Could you check a few things on this model? Use its own coordinates, in mm. Give positions to 0.01 mm unless a question says otherwise; leave off trailing zeros. Order: outer loops, then holes, each group sorted by start corner. A loop starts at its lowest first (then second) coordinate and runs counter-clockwise, first axis right, second up. Notation, with made-up numbers: M 57,-16 L 107,-16 A22 cw 107,0 Z; hole C 29.25,21 d10. An arc over 180 degrees is marked long. Answer in a Markdown table with one row per item. Add a question column.
```python
from build123d import *

# Parameters (mm, degrees)
EXTRUDE_1_DEPTH          = 3
SKETCH_2_R               = 37.6
CUT_EXTRUDE_1_DEPTH      = 3
SKETCH_1_4_R             = 2.7
CUT_EXTRUDE_5_DEPTH      = 10
PATTERN_CIRCULAR_2_COUNT = 4


with BuildPart() as part:
    # Sketch 1 → Extrude 1 (new body)
    with BuildSketch(Plane(origin=(0, 0, 0), x_dir=(1, 0, 0), z_dir=(0, 1, 0))):
        with BuildLine():
            Line((-49, 45), (-49, -45))
            ThreePointArc((-49, -45), (-47.828427125, -47.828427125), (-45, -49))
            Line((-45, -49), (45, -49))
            ThreePointArc((45, -49), (47.828427125, -47.828427125), (49, -45))
            Line((49, -45), (49, 45))
            ThreePointArc((49, 45), (47.828427125, 47.828427125), (45, 49))
            Line((45, 49), (-45, 49))
            ThreePointArc((-45, 49), (-47.828427125, 47.828427125), (-49, 45))
        make_face()
    extrude(amount=EXTRUDE_1_DEPTH)

    # Sketch 2 → Cut-Extrude 1 (cut)
    with BuildSketch(Plane(origin=(0, 3, 0), x_dir=(1, 0, 0), z_dir=(0, 1, 0))):
        with Locations(Location((0, 0, 0), (0, 0, 270))):
            Circle(SKETCH_2_R)
    extrude(amount=-CUT_EXTRUDE_1_DEPTH, mode=Mode.SUBTRACT)

    # Sketch 1_4 → Cut-Extrude 5 (cut)
    with BuildSketch(Plane(origin=(0, 0, 0), x_dir=(1, 0, 0), z_dir=(0, 1, 0))):
        with Locations(Location((45, -45, 0), (0, 0, 270))):
            Circle(SKETCH_1_4_R)
    cut_extrude_5 = extrude(amount=CUT_EXTRUDE_5_DEPTH, mode=Mode.SUBTRACT)

    # Pattern Circular 2: Cut-Extrude 5 ×4 about axis
    pattern_circular_2_axis = Axis((0, 0, 0), (0, 1, 0))
    for i in range(1, PATTERN_CIRCULAR_2_COUNT):
        add(cut_extrude_5.rotate(pattern_circular_2_axis, i * 360 / PATTERN_CIRCULAR_2_COUNT), mode=Mode.SUBTRACT)


solid = part.part
```
1. Suppose I cut it at A-A on y = 1.1. List the corners of the cut face in (x, z) for me, plus the area to 3 significant figures.
2. Suppose I cut it at C-C on x = 0. List the corners of the cut face in (y, z) for me.
3. Suppose I cut it at B-B on z = 0. List the corners of the cut face in (x, y) for me, plus the area to 3 significant figures.
4. If I drill on line 1 along Z through (x, y) = (45, 1.45); line 2 along Z through (x, y) = (0.5, 0.25), over which ranges is the centre line in solid material (lowest first)? Write a range as [from, to].
5. Thinking about a two-plate mould opening in X: for faces 1 (the flat face through (-1, 1, 49)), 2 (the flat face through (-49, 1, -1)), 3 (the cylindrical face through (-47.575, 1.479, 45.811)), 4 (the cylindrical face through (47.859, 1.479, -47.797)), which applies, pulls with the +X half, pulls with the -X half, needs draft (parallel to the pull), parting line crosses it, or undercut?
6. Will these pins go through, and if not, where does the flat tip stop? P1, Ø10, axis at x = 34.5, z = 12, coming from the +Y side; P2, Ø4.5, axis at x = -45, z = -45, coming from the +Y side.
Findings below:
| question | item | result |
|---|---|---|
| 1 | outline | M -49,-45 A4 ccw -45,-49 L 45,-49 A4 ccw 49,-45 L 49,45 A4 ccw 45,49 L -45,49 A4 ccw -49,45 Z; hole C -45,-45 d5.4; hole C -45,45 d5.4; hole C 0,0 d75.2; hole C 45,-45 d5.4; hole C 45,45 d5.4 |
| 1 | area | 5,060 mm2 |
| 2 | outline | M 0,-49 L 3,-49 L 3,-37.6 L 0,-37.6 Z; M 0,37.6 L 3,37.6 L 3,49 L 0,49 Z |
| 3 | outline | M -49,0 L -37.6,0 L -37.6,3 L -49,3 Z; M 37.6,0 L 49,0 L 49,3 L 37.6,3 Z |
| 3 | area | 68.4 mm2 |
| 4 | line 1 | [-49, -47.7], [-42.3, 42.3], [47.7, 49] |
| 4 | line 2 | [-49, -37.6], [37.6, 49] |
| 5 | face 1 | needs draft |
| 5 | face 2 | pulls with the -X half |
| 5 | face 3 | undercut |
| 5 | face 4 | pulls with the +X half |
| 6 | P1 | y = 3 |
| 6 | P2 | through |
